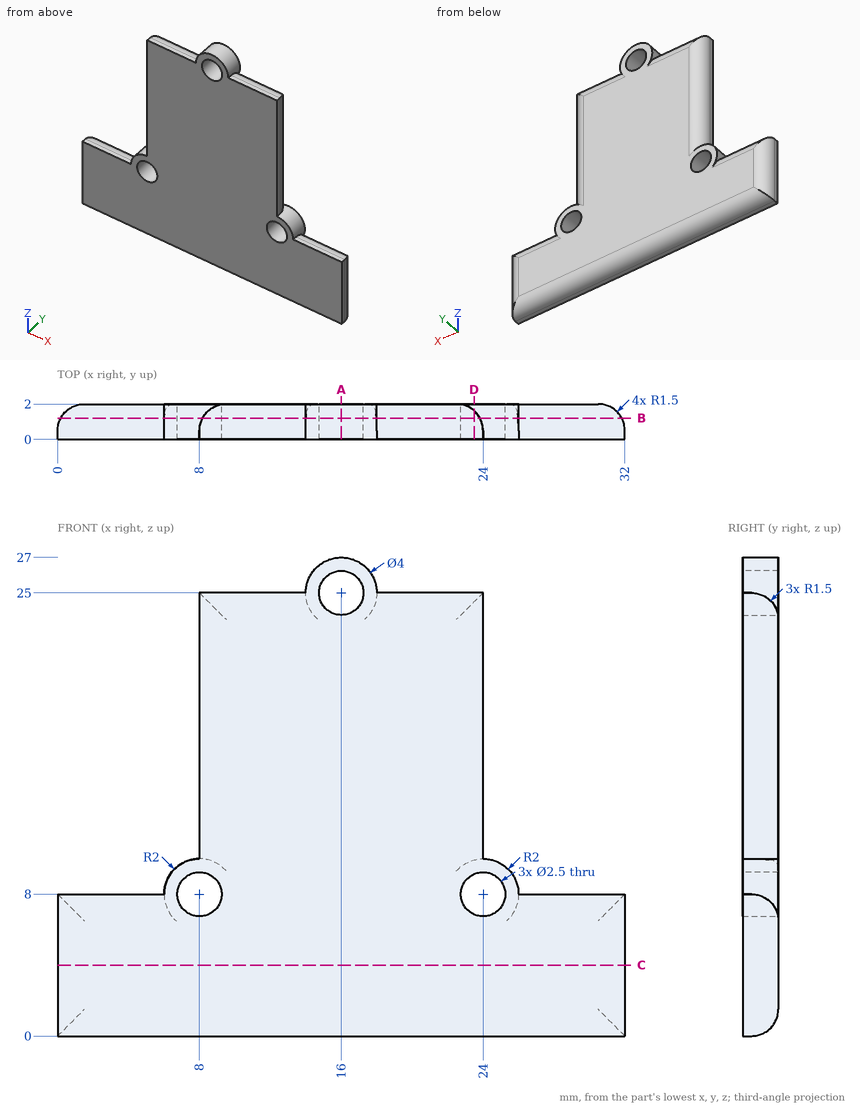
Could you check a few things on this drawing? It's one solid part, dimensions in mm from its lowest x, y, z. Give positions to 0.01 mm unless a question says otherwise; leave off trailing zeros. Loops run counter-clockwise (first coordinate to the right, second up) from the corner with the lowest first, then second, coordinate; pieces in that order, holes last. Notation, with made-up numbers: (-18, 71) -> (-11, 71) arc R35 cw to (-11, 110) -> close; hole circle Ø1 at (51, -22.5). An arc over 180 degrees is marked (long way). Answer as CSV lines item,"result". Start each with the question number.
(1) If we section it at B-B on y = 1.2: Write out the boundary of the cut face in (x, z).
(2) I'm going to push flat-ended pins straight in: pin 1 Ø1 at (y, z) = (0, 11.5) entering from +X; pin 2 Ø1.5 at (x, z) = (23.5, 23) entering from +Y; pin 3 Ø0.6 at (y, z) = (0, 18) entering from -X. Where does each tip first touch, or does it pass through?
(3) If we section it at D-D on x = 23.5: Write out the boundary of the cut face in (y, z), then the cut area to 3 significant figures.
(4) If we section it at C-C on z = 4: Write out the boundary of the cut face in (x, y), then the cut area to 3 significant figures.
(5) If we section it at A-A on x = 16: Write out the boundary of the cut face in (y, z).
(6) I need wall thicknesses on probe 1 along X at (y, z) = (0.95, 8); probe 2 along X at (y, z) = (0.65, 6.25); probe 3 along X at (y, z) = (0.9, 25). Which ranges of each line are inside material? Lowest first, please.
Computed:
1,outline,"(0.17, 0.17) -> (31.83, 0.17) -> (31.83, 7.83) -> (25.99, 7.83) arc R2 ccw to (23.83, 9.99) -> (23.83, 24.83) -> (17.99, 24.83) arc R2 ccw (long way) to (14.01, 24.83) -> (8.17, 24.83) -> (8.17, 9.99) arc R2 ccw to (6.01, 7.83) -> (0.17, 7.83) -> close; hole circle Ø2.5 at (8, 8); hole circle Ø2.5 at (16, 25); hole circle Ø2.5 at (24, 8)"
2,pin 1,"stops at x = 24"
2,pin 2,"stops at y = 1.98"
2,pin 3,"stops at x = 8"
3,outline,"(0, 0) -> (0.5, 0) arc R1.5 ccw to (2, 1.5) -> (2, 6.85) -> (0, 6.85) -> close; (0, 9.15) -> (2, 9.15) -> (2, 9.94) -> (1.62, 9.94) -> (1.62, 24.5) arc R1.5 ccw to (0.5, 25) -> (0, 25) -> close"
3,area,"39.0 mm2"
4,outline,"(0, 0) -> (32, 0) -> (32, 0.5) arc R1.5 ccw to (30.5, 2) -> (1.5, 2) arc R1.5 ccw to (0, 0.5) -> close"
4,area,"63.0 mm2"
5,outline,"(0, 0) -> (0.5, 0) arc R1.5 ccw to (2, 1.5) -> (2, 23.75) -> (0, 23.75) -> close; (0, 26.25) -> (2, 26.25) -> (2, 27) -> (0, 27) -> close"
6,probe 1,"x = 6 to 6.75, 9.25 to 22.75, 25.25 to 26"
6,probe 2,"x = 0.01 to 31.99"
6,probe 3,"x = 14 to 14.75, 17.25 to 18"
